Can you work these out from the model? Positions are in its coordinate system, mm. Face numbers are marked on the shaded views. A direction names the side the tool comes from. Coordinates: 2 decimals unless noted, no trailing zeros. Loops run counter-clockwise (first coordinate to the right, second up) from the corner with the lowest first, then second, coordinate; pieces in that order, holes last.
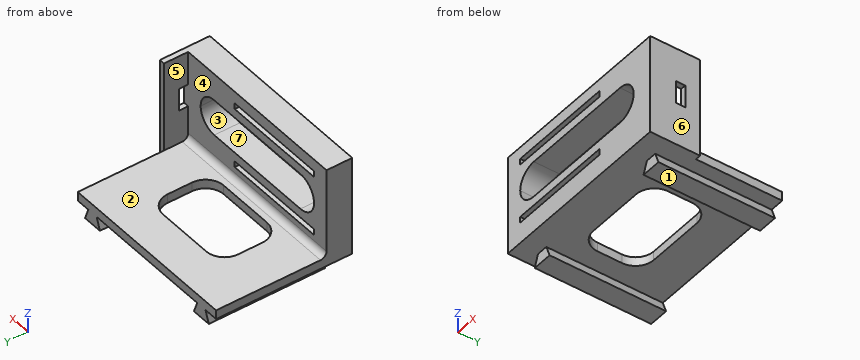
```python
from build123d import *

# Parameters (mm, degrees)
SKETCH1_W           = 61
SKETCH1_H           = 45
BOSS_EXTRUDE1_DEPTH = 3
BOSS_EXTRUDE2_DEPTH = 38.5
SKETCH3_W           = 61
SKETCH3_H           = 30
BOSS_EXTRUDE3_DEPTH = 8.5
SKETCH4_W           = 35
SKETCH4_H           = 2
CUT_EXTRUDE1_DEPTH  = 8.5
SKETCH5_W           = 33
SKETCH5_H           = 16.5
SKETCH5_W_2         = 7.5
SKETCH5_H_2         = 3.1
BOSS_EXTRUDE4_DEPTH = 1.8
CUT_EXTRUDE2_REACH  = 60.86
SKETCH6_W           = 50
SKETCH6_H           = 12
CUT_EXTRUDE3_REACH  = 53.367
SKETCH7_W           = 31
SKETCH7_H           = 20
FILLET1_R           = 6
FILLET2_R           = 2


with BuildPart() as part:
    # Sketch1 → Boss-Extrude1 (new body)
    with BuildSketch(Plane.XY):
        Rectangle(SKETCH1_W, SKETCH1_H)
    extrude(amount=BOSS_EXTRUDE1_DEPTH)

    # Sketch2 → Boss-Extrude2 (add)
    with BuildSketch(Plane(origin=(0, 22.5, 0), x_dir=(1, 0, 0), z_dir=(0, 1, 0))):
        Polygon((-25.83979993, 0), (-27.28354993, 3.85), (-20.71645007, 3.85), (-22.16020007, 0), align=None)
        Polygon((20.71645007, 3.85), (22.16020007, 0), (25.83979993, 0), (27.28354993, 3.85), align=None)
    extrude(amount=-BOSS_EXTRUDE2_DEPTH)

    # Sketch3 → Boss-Extrude3 (add)
    with BuildSketch(Plane.XZ.offset(22.5)):
        with Locations((0, 18)):
            Rectangle(SKETCH3_W, SKETCH3_H)
    extrude(amount=-BOSS_EXTRUDE3_DEPTH)

    # Sketch4 → Cut-Extrude1 (cut)
    with BuildSketch(Plane(origin=(0, -14, 0), x_dir=(1, 0, 0), z_dir=(0, 1, 0))):
        with Locations((-7.5, -8)):
            Rectangle(SKETCH4_W, SKETCH4_H)
        with Locations((-7.5, -28)):
            Rectangle(SKETCH4_W, SKETCH4_H)
    extrude(amount=-CUT_EXTRUDE1_DEPTH, mode=Mode.SUBTRACT)

    # Sketch5 → Boss-Extrude4 (add)
    with BuildSketch(Plane(origin=(30.5, 0, 0), x_dir=(0, 0, -1), z_dir=(1, 0, 0))):
        with Locations((-16.5, -14.25)):
            Rectangle(SKETCH5_W, SKETCH5_H)
        with Locations((-18, -12.45)):
            Rectangle(SKETCH5_W_2, SKETCH5_H_2, mode=Mode.SUBTRACT)
    extrude(amount=BOSS_EXTRUDE4_DEPTH)

    # Sketch6 → Cut-Extrude2 (cut, up to next)
    with BuildSketch(Plane(origin=(0, -14, 0), x_dir=(1, 0, 0), z_dir=(0, 1, 0)), mode=Mode.PRIVATE) as cut_extrude2_sk1:
        with Locations((0, -18)):
            Rectangle(SKETCH6_W, SKETCH6_H)
    cut_extrude2_tool1 = extrude(cut_extrude2_sk1.sketch, amount=-CUT_EXTRUDE2_REACH, mode=Mode.PRIVATE) & part.part
    add(cut_extrude2_tool1.solids().sort_by_distance((0, -14, 18))[0], mode=Mode.SUBTRACT)

    # Sketch7 → Cut-Extrude3 (cut, up to next)
    with BuildSketch(Plane(origin=(0, 0, 0), x_dir=(-1, 0, 0), z_dir=(0, 0, -1)), mode=Mode.PRIVATE) as cut_extrude3_sk1:
        Rectangle(SKETCH7_W, SKETCH7_H)
    cut_extrude3_tool1 = extrude(cut_extrude3_sk1.sketch, amount=-CUT_EXTRUDE3_REACH, mode=Mode.PRIVATE) & part.part
    add(cut_extrude3_tool1.solids().sort_by_distance((0, 0, 0))[0], mode=Mode.SUBTRACT)

    # Fillet1
    fillet1_edges = [part.edges().sort_by_distance(p)[0] for p in [
        (-25, -18.25, 24),
        (-25, -18.25, 12),
        (25, -18.25, 24),
        (25, -18.25, 12),
        (-15.5, -10, 1.5),
        (-15.5, 10, 1.5),
        (15.5, 10, 1.5),
        (15.5, -10, 1.5),
    ]]
    fillet(fillet1_edges, radius=FILLET1_R - 0.0001)  # a hair under: the kernel refuses the full size

    # Fillet2
    fillet2_edges = [part.edges().sort_by_distance(p)[0] for p in [
        (0, -14, 3),
    ]]
    fillet(fillet2_edges, radius=FILLET2_R)


solid = part.part
```
(1) I want a section at A-A on y = 3. Write out the boundary of the cut face in (x, z).
Check values:
outline: (-30.5, 0) - (-25.84, 0) - (-27.28, -3.85) - (-20.72, -3.85) - (-22.16, 0) - (-15.5, 0) - (-15.5, 3) - (-30.5, 3) - close; (15.5, 0) - (22.16, 0) - (20.72, -3.85) - (27.28, -3.85) - (25.84, 0) - (30.5, 0) - (30.5, 3) - (15.5, 3) - close
(2) Which directions (+Z, -Z, +X, -X, +Y, -Y) give clear straight access to the entire face, cutting with the end or side of a thin tool? Please do the marked faces 1, 2 and 3.
Check values:
face 1: -Z, +X, -X, +Y, -Y
face 2: +Z, -X, +Y
face 3: +Y, -Y
(3) I'm going to push flat-ended pins straight in: pin 1 (1.2 mm diameter, centred on x = 24.5, z = -1.5, fed in from -Y); pin 2 (9.5 mm diameter, centred on x = -16, y = -17, fed in from -Z); pin 3 (4 mm diameter, centred on y = -11.5, z = 25, fed in from -X). Where does each tip first touch, or does it pass through?
Check values:
pin 1: stops at y = -16
pin 2: stops at z = 0
pin 3: stops at x = 30.5
(4) I want a section at C-C on y = -15. State how many separate pieces and enclosed holes the cut face has, then the cut area to 3 significant figures.
Check values:
separate pieces: 1
enclosed holes: 3
area: 1,400 mm2
(5) If I drill on probe 1 along Z at (x, y) = (-21, -20); probe 2 along Y at (x, z) = (28, 11); probe 3 along Z at (x, y) = (27.5, 15.5), over which ranges is the centre line in solid material (lowest first)?
Check values:
probe 1: z = 0 to 7, 9 to 12.34, 23.66 to 27, 29 to 33
probe 2: y = -22.5 to -14
probe 3: z = 0 to 3
(6) I want a section at D-D on x = -8.5. Write out the boundary of the cut face in (y, z), then the cut area to 3 significant figures.
Check values:
outline: (-22.5, 0) - (-10, 0) - (-10, 3) - (-12, 3) arc R2 cw to (-14, 5) - (-14, 7) - (-22.5, 7) - close; (-22.5, 9) - (-14, 9) - (-14, 12) - (-22.5, 12) - close; (-22.5, 24) - (-14, 24) - (-14, 27) - (-22.5, 27) - close; (-22.5, 29) - (-14, 29) - (-14, 33) - (-22.5, 33) - close; (10, 0) - (22.5, 0) - (22.5, 3) - (10, 3) - close
area: 195 mm2
(7) If we mould it in two halves opening along X, with no side actions, what happens to the marked faces 4, 5, 6 and 7? For each: released by +X, released by -X, zero draft, split by the parting line, or undercut.
Check values:
face 4: zero draft
face 5: released by -X
face 6: released by +X
face 7: undercut
(8) I want a section at B-B on z = 1.5. Write out the boundary of the cut face in (x, y).
Check values:
outline: (-30.5, -22.5) - (32.3, -22.5) - (32.3, -6) - (30.5, -6) - (30.5, 22.5) - (-30.5, 22.5) - close; hole (-15.5, -4) arc R6 ccw to (-9.5, -10) - (9.5, -10) arc R6 ccw to (15.5, -4) - (15.5, 4) arc R6 ccw to (9.5, 10) - (-9.5, 10) arc R6 ccw to (-15.5, 4) - close
